```python
from build123d import *
from build123d.topology import SkipClean

# Parameters (mm, degrees)
SKETCH_1_W          = 29.5
SKETCH_1_H          = 13
EXTRUDE_1_DEPTH     = 13.5
EXTRUDE_2_DEPTH     = 2
SKETCH_3_W          = 7.5
SKETCH_3_H          = 7.5
SKETCH_3_W_2        = 16.3
CUT_EXTRUDE_1_DEPTH = 6
SKETCH_7_W          = 10.1
SKETCH_7_H          = 3.3
EXTRUDE_3_DEPTH     = 6


with BuildPart() as part:
    # Sketch 1 → Extrude 1 (new body)
    with BuildSketch(Plane.XY):
        Rectangle(SKETCH_1_W, SKETCH_1_H)
    extrude(amount=EXTRUDE_1_DEPTH)

    # Sketch 2 → Extrude 2 (add)
    with BuildSketch(Plane(origin=(0, 0, 0), x_dir=(-1, 0, 0), z_dir=(0, 0, -1))):
        Polygon((-14.75, 0), (-14.75, -3.75), (14.75, -3.75), (14.75, 0), (14.75, 3.75), (-14.75, 3.75), align=None)
        with BuildLine():
            Line((-14.75, 3.75), (-18.5, 3.75))
            ThreePointArc((-18.5, 3.75), (-15.848349571, 2.651650429), (-14.75, 0))
            Line((-14.75, 0), (-14.75, 3.75))
        make_face()
        with BuildLine():
            ThreePointArc((-18.5, 3.75), (-22.25, 0), (-18.5, -3.75))
            Line((-18.5, -3.75), (-18.5, -1.6))
            ThreePointArc((-18.5, -1.6), (-20.1, 0), (-18.5, 1.6))
            Line((-18.5, 1.6), (-18.5, 3.75))
        make_face()
        with BuildLine():
            Line((-18.5, -1.6), (-18.5, -3.75))
            ThreePointArc((-18.5, -3.75), (-15.848349571, -2.651650429), (-14.75, 0))
            ThreePointArc((-14.75, 0), (-15.848349571, 2.651650429), (-18.5, 3.75))
            Line((-18.5, 3.75), (-18.5, 1.6))
            ThreePointArc((-18.5, 1.6), (-17.36862915, 1.13137085), (-16.9, 0))
            ThreePointArc((-16.9, 0), (-17.36862915, -1.13137085), (-18.5, -1.6))
        make_face()
        with BuildLine():
            ThreePointArc((-14.75, 0), (-15.848349571, -2.651650429), (-18.5, -3.75))
            Line((-18.5, -3.75), (-14.75, -3.75))
            Line((-14.75, -3.75), (-14.75, 0))
        make_face()
        with BuildLine():
            Line((14.75, 3.75), (14.75, 0))
            ThreePointArc((14.75, 0), (15.848349571, 2.651650429), (18.5, 3.75))
            Line((18.5, 3.75), (14.75, 3.75))
        make_face()
        with BuildLine():
            Line((14.75, 0), (14.75, -3.75))
            Line((14.75, -3.75), (18.5, -3.75))
            ThreePointArc((18.5, -3.75), (15.848349571, -2.651650429), (14.75, 0))
        make_face()
        with BuildLine():
            ThreePointArc((14.75, 0), (15.848349571, -2.651650429), (18.5, -3.75))
            Line((18.5, -3.75), (18.5, -1.6))
            ThreePointArc((18.5, -1.6), (16.9, 0), (18.5, 1.6))
            Line((18.5, 1.6), (18.5, 3.75))
            ThreePointArc((18.5, 3.75), (15.848349571, 2.651650429), (14.75, 0))
        make_face()
        with BuildLine():
            Line((18.5, -1.6), (18.5, -3.75))
            ThreePointArc((18.5, -3.75), (21.151650429, -2.651650429), (22.25, 0))
            ThreePointArc((22.25, 0), (21.151650429, 2.651650429), (18.5, 3.75))
            Line((18.5, 3.75), (18.5, 1.6))
            ThreePointArc((18.5, 1.6), (19.63137085, 1.13137085), (20.1, 0))
            ThreePointArc((20.1, 0), (19.63137085, -1.13137085), (18.5, -1.6))
        make_face()
    extrude(amount=-EXTRUDE_2_DEPTH)

    # Sketch 3 → Cut-Extrude 1 (cut)
    with BuildSketch(Plane.XY.offset(13.5)):
        with Locations((-10.25, 0)):
            Rectangle(SKETCH_3_W, SKETCH_3_H)
        with Locations((5.8, 0)):
            Rectangle(SKETCH_3_W_2, SKETCH_3_H)
    extrude(amount=-CUT_EXTRUDE_1_DEPTH, mode=Mode.SUBTRACT)

    # Sketch 4 → Revolve 1 (revolve)
    with BuildSketch(Plane.XY.offset(7.5)):
        with BuildLine():
            Line((-10.25, 3.75), (-10.25, -3.75))
            ThreePointArc((-10.25, -3.75), (-14, 0), (-10.25, 3.75))
        make_face()
    revolve(axis=Axis((-10.25, 3.75, 7.5), (0, -1, 0)))

    # Sketch 6 → Revolve 14 (revolve)
    with SkipClean():  # the faces are left unmerged after this step: merging them gives an invalid solid
        with BuildSketch(Plane.XY.offset(7.5)):
            with BuildLine():
                ThreePointArc((9.902834279, 3.75), (6.152834279, 0), (9.902834279, -3.75))
                Line((9.902834279, -3.75), (9.902834279, 3.75))
            make_face()
            with BuildLine():
                Line((9.902834279, 3.75), (9.902834279, -3.75))
                ThreePointArc((9.902834279, -3.75), (12.554484709, -2.651650429), (13.652834279, 0))
                ThreePointArc((13.652834279, 0), (12.554484709, 2.651650429), (9.902834279, 3.75))
            make_face()
        revolve(axis=Axis((9.902834279, -3.75, 7.5), (0, 1, 0)))
    add(part.part.scale(1), mode=Mode.REPLACE)  # the faces are merged on a copy

    # Sketch 7 → Extrude 3 (add)
    with BuildSketch(Plane.XZ.offset(6.5)):
        with Locations((1, 1.65)):
            Rectangle(SKETCH_7_W, SKETCH_7_H)
    extrude(amount=EXTRUDE_3_DEPTH)


solid = part.part
```
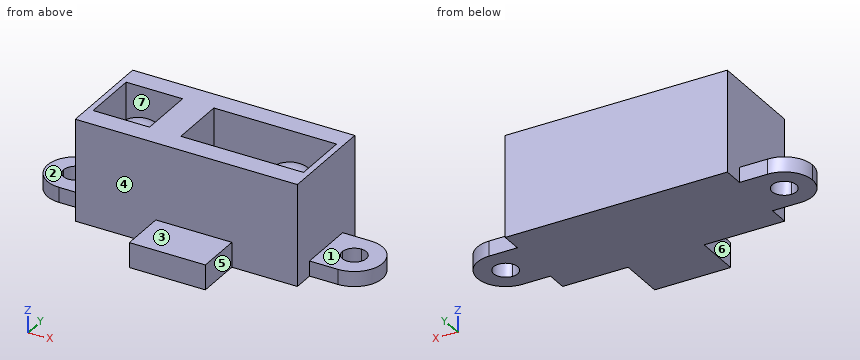
CAD build for the part. Positions are in the model's coordinates, mm. Face numbers are marked on the shaded views. A direction names the side the tool comes from. Give positions to 0.01 mm unless a question says otherwise; leave off trailing zeros. Loops run counter-clockwise (first coordinate to the right, second up) from the corner with the lowest first, then second, coordinate; pieces in that order, holes last. Notation, with made-up numbers: M 11,-3.75 L 51,-3.75 A22 ccw 51,9.25 Z; hole C -36,-14.75 d7. An arc over 180 degrees is marked long. Use one line per item in the form item = value.
Item 1: Slice it at C-C (y = -5.25). List the corners of the cut face in (x, z), plus the area to 3 significant figures.
Determined:
outline = M -14.75,0 L 14.75,0 L 14.75,13.5 L -14.75,13.5 Z
area = 398 mm2
Item 2: Drill centre lines: probe 1 along Y at (x, z) = (3, 12); probe 2 along X at (y, z) = (1.5, 8.5); probe 3 along Y at (x, z) = (-2, 5). Where is each one in solid material? Low to high. Write a range as from..to.
Determined:
probe_1 = -6.5..-3.75, 3.75..6.5
probe_2 = -14.75..-14, -13.54..-6.96, -6.5..-2.35, 6.61..13.19, 13.95..14.75
probe_3 = -6.5..6.5
Item 3: Which spindle directions (+Z, -Z, +X, -X, +Y, -Y) get a long thin tool onto all of the face, cutting with end or side? Do the marked faces 1, 2 and 3. Say none if no direction does.
Determined:
face_1 = +Z, +X, +Y, -Y
face_2 = +Z, -X, +Y, -Y
face_3 = +Z, +X, -X, -Y
Item 4: Slice it at B-B (x = 18). List the corners of the cut face in (y, z), plus the area to 3 significant figures.
Determined:
outline = M -3.75,0 L -1.52,0 L -1.52,2 L -3.75,2 Z; M 1.52,0 L 3.75,0 L 3.75,2 L 1.52,2 Z
area = 8.92 mm2
Item 5: Slice it at D-D (x = -16). List the corners of the cut face in (y, z).
Determined:
outline = M -3.75,0 L 3.75,0 L 3.75,2 L -3.75,2 Z
Item 6: Flat gauge pins, fed straight in: pin 1 (3 mm diameter, centred on y = -0.5, z = 11.5, fed in from -X); pin 2 (6 mm diameter, centred on x = 16.5, z = 11, fed in from -Y); pin 3 (1.1 mm diameter, centred on x = -12, y = 1.5, fed in from +Z). Where does each tip first touch, or does it go through?
Determined:
pin_1 = -14.75
pin_2 = -6.5
pin_3 = 10.81
Item 7: Two-plate mould, pull along X, no slides. Class the marked faces 4, 5, 6 and 7: pulls with the +X half, pulls with the -X half, needs draft (parallel to the pull), parting line crosses it, or undercut.
Determined:
face_4 = needs draft
face_5 = pulls with the +X half
face_6 = pulls with the -X half
face_7 = undercut
Item 8: Slice it at A-A (z = 10). List the corners of the cut face in (x, y).
Determined:
outline = M -14.75,-6.5 L 14.75,-6.5 L 14.75,6.5 L -14.75,6.5 Z; C -10.25,0 d5.59; C 9.9,0 d5.59; hole M -14,-3.75 L -6.5,-3.75 L -6.5,3.75 L -14,3.75 Z; hole M -2.35,-3.75 L 13.95,-3.75 L 13.95,3.75 L -2.35,3.75 Z
